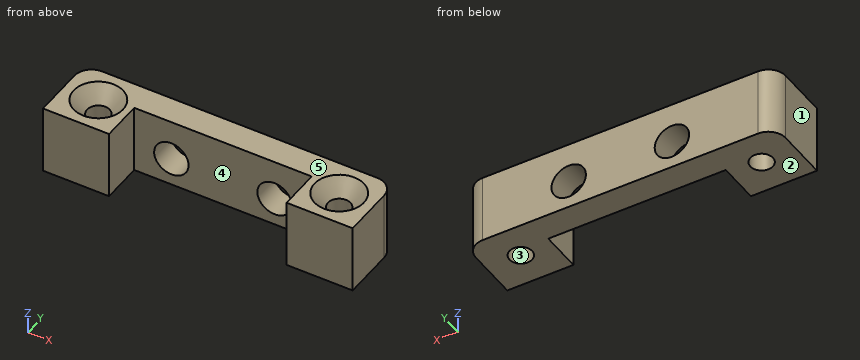
Solid Edge part; units mm, degrees
sketch "Sketch1" plane through (0, 0, 0) normal (0, -1, 0) x (1, 0, 0)
  line L0 (0, 0) -> (0, 12.7)
  line L1 (0, 12.7) -> (57.15, 12.7)
  line L2 (57.15, 12.7) -> (57.15, 0)
  line L3 (57.15, 0) -> (0, 0)
  dimension "D1" = 57.15
extrude "Protrusion1" add sketch "Sketch1" against normal blind 12.7
sketch "Sketch2" plane through (39.624, 0, 4.7625) normal (0, -1, 0) x (1, 0, 0)
  line L0 (-27.432, -4.7625) -> (-27.432, 7.9375)
  line L1 (-27.432, 7.9375) -> (5.334, 7.9375)
  line L2 (5.334, 7.9375) -> (5.334, -4.7625)
  line L3 (5.334, -4.7625) -> (-27.432, -4.7625)
extrude "ExtrudedCutout_3" cut sketch "Sketch2" against normal blind 7.62
hole "Hole_13" at (50.8, 6.35, 12.7) direction (0, 0, -1) diameter 4.1656 end up to next countersink diameter 9.1186 countersink angle 82
hole "Hole1" at (6.35, 6.35, 12.7) direction (0, 0, -1) diameter 4.1656 end up to next countersink diameter 9.1186 countersink angle 82
hole "Hole_11" at (19.05, 12.7, 5.2324) direction (0, -1, 0) diameter 6.35 end up to next
hole "Hole2" at (38.1, 12.7, 5.2324) direction (0, -1, 0) diameter 6.35 end up to next
fillet "Round_1" radius 3.175 2 edges at (57.15, 12.7, 6.35) (0, 12.7, 6.35)
properties material "Polyethylene, low density"
Geometry: final body of the model. Coordinates: model frame, mm. Face numbers are marked on the shaded views. A direction names the side the tool comes from. Coordinates: 2 decimals unless noted, no trailing zeros. Order: outer loops, then holes, each group sorted by start corner. A loop starts at its lowest first (then second) coordinate and runs counter-clockwise, first axis right, second up. Notation, with made-up numbers: (-37.75, 53) - (-26.75, 53) arc R28 cw to (-26.75, 83) - close; hole circle Ø5 at (53, 17.25). An arc over 180 degrees is marked (long way). Return JSON: item names as keys, results as strings. Group by question number.
1. Pull-direction query (X, two-part tool) for the marked faces 1, 2 and 3; classes: pulls with the +X half, pulls with the -X half, needs draft (parallel to the pull), parting line crosses it, or undercut.
2. Cut plane B-B (y = 6.35). Output: boundary loops of the cut face in (x, z).
3. Cut plane D-D (y = 1). Output: boundary loops of the cut face in (x, z), plus the area to 3 significant figures.
4. Material intervals for line 1 along X through (y, z) = (6.35, 4); line 2 along Z through (x, y) = (19.05, 9.5); line 3 along X through (y, z) = (12, 6), sorted ascending. Write a range as [from, to].
5. Cut plane A-A (x = 38.1). Output: boundary loops of the cut face in (y, z).
6. Cut plane C-C (z = 5.75). Output: boundary loops of the cut face in (x, y) (3 decimals), plus the area to 3 significant figures.
7. Set-up query: the marked faces 4 and 5. Return all of +Z, -Z, +X, -X, +Y, -Y with unobstructed straight access to the full face (end or side cutting, diameter ignored); none if empty.
8. Pin query (flat end, axial travel): pin 1 (4 mm diameter, centred on x = 29, y = 10.5, fed in from -Z); pin 2 (6.5 mm diameter, centred on x = 35.5, z = 8.5, fed in from -Y); pin 3 (4 mm diameter, centred on x = 38.1, z = 5.23, fed in from +Y). Return the tip coordinate at first contact, or that it passes through.
Resolved:
{
 "1": {"face 1": "pulls with the -X half", "face 2": "needs draft", "face 3": "undercut"},
 "2": {"outline": "(0, 0) - (4.27, 0) - (4.27, 9.85) - (1.79, 12.7) - (0, 12.7) - close; (8.43, 0) - (12.19, 0) - (12.19, 12.7) - (10.91, 12.7) - (8.43, 9.85) - close; (44.96, 0) - (48.72, 0) - (48.72, 9.85) - (46.24, 12.7) - (44.96, 12.7) - close; (52.88, 0) - (57.15, 0) - (57.15, 12.7) - (55.36, 12.7) - (52.88, 9.85) - close"},
 "3": {"outline": "(0, 0) - (12.19, 0) - (12.19, 12.7) - (0, 12.7) - close; (44.96, 0) - (57.15, 0) - (57.15, 12.7) - (44.96, 12.7) - close", "area": "310 mm²"},
 "4": {"line 1": "x = [0, 4.27], [8.43, 12.19], [44.96, 48.72], [52.88, 57.15]", "line 2": "z = [0, 2.06], [8.41, 12.7]", "line 3": "x = [1.19, 15.97], [22.13, 35.02], [41.18, 55.96]"},
 "5": {"outline": "(7.62, 0) - (12.7, 0) - (12.7, 2.06) - (7.62, 2.06) - close; (7.62, 8.41) - (12.7, 8.41) - (12.7, 12.7) - (7.62, 12.7) - close"},
 "6": {"outline": "(0, 0) - (12.192, 0) - (12.192, 7.62) - (15.917, 7.62) - (15.917, 12.7) - (3.175, 12.7) arc R3.175 ccw to (0, 9.525) - close; (22.183, 7.62) - (34.967, 7.62) - (34.967, 12.7) - (22.183, 12.7) - close; (41.233, 7.62) - (44.958, 7.62) - (44.958, 0) - (57.15, 0) - (57.15, 9.525) arc R3.175 ccw to (53.975, 12.7) - (41.233, 12.7) - close; hole circle Ø4.166 at (6.35, 6.35); hole circle Ø4.166 at (50.8, 6.35)", "area": "381 mm²"},
 "7": {"face 4": "+Z, -Z, -Y", "face 5": "+Z, +X, -X, +Y, -Y"},
 "8": {"pin 1": "stops at z = 0", "pin 2": "stops at y = 7.62", "pin 3": "passes through"}
}
